The model under review builds one solid part; all positions refer to its coordinate system, in mm. A direction names the side the tool comes from. Coordinates: 2 decimals unless noted, no trailing zeros. Loops run counter-clockwise (first coordinate to the right, second up) from the corner with the lowest first, then second, coordinate; pieces in that order, holes last. Notation, with made-up numbers: M -9,12 L 42,12 A15 ccw 42,32 Z; hole C -4.75,-14.5 d1. An arc over 180 degrees is marked long. Write item = value, one per line. Start each with the question number.
Q1. For faces 5 (the face through (6.847, -0.766, -6.591)), 6 (the face through (3, 0, 0)), 7 (the face through (-5, 0, 5)), 8 (the face through (40, -5, -2)), 9 (the face through (-5, 0, -5)), list the 3-axis set-ups (+Z, -Z, +X, -X, +Y, -Y) from which the entire face can be reached by the end or side of a thin tool; tool diameter is ignored.
Q2. Mouldability with a two-part tool opening along Y and no side actions: class faces 1 (the face through (39.01, -4.88, 1.08)), 2 (the face through (19.72, -2.87, -6.93)), 3 (the face through (0, 2, 2)), 4 (the face through (38, 4, 4)) as released by +Y, released by -Y, zero draft, split by the parting line, or undercut.
Q3. Clearance check with flat-ended pins moving along their axes: pin 1 Ø1 at (x, y) = (16, -1) entering from -Z; pin 2 Ø5.5 at (x, y) = (-5.5, -1) entering from +Z; pin 3 Ø4 at (x, y) = (-5.5, -1) entering from -Z. State where each tip first meets the part, or that it passes through.
Q4. We need section A-A on y = 1.25. Give the boundary of the cut face in (x, z), and give its area (3 significant figures).
Q5. We need section D-D on x = 14. Give the boundary of the cut face in (y, z), and give its area (3 significant figures).
Q6. Wall thickness on probe 1 along X at (y, z) = (5, 2.5); probe 2 along Y at (x, z) = (38.75, 0); probe 3 along X at (y, z) = (-3.25, 6.25): over which ranges is each line inside the solid? List them lowest first.
Q7. We need section B-B on x = 5. Give the boundary of the cut face in (y, z).
Q8. We need section C-C on z = 0. Give the boundary of the cut face in (x, y), and give its area (3 significant figures).
from build123d import *

# Parameters (mm, degrees)
SKETCH1_R                = 7.5
BOSS_EXTRUDE1_DEPTH      = 40
SKETCH2_R                = 5
CUT_EXTRUDE1_DEPTH       = 2
SKETCH3_R                = 6
CUT_EXTRUDE2_DEPTH       = 35
SKETCH4_R                = 2.5
BOSS_EXTRUDE4_DEPTH      = 5
BOSS_EXTRUDE5_DEPTH      = 5
BOSS_EXTRUDE5_DEPTH_BACK = 5
SKETCH6_R                = 2.5
CUT_EXTRUDE3_START       = -7.500000101
CUT_EXTRUDE3_OUTLINE_R   = 2
CUT_EXTRUDE3_DEPTH       = 15.000000201


# Read off the part's stored shape, not the designer's step: Cut-Extrude3
with BuildPart() as part:
    # Sketch1 → Boss-Extrude1 (new body)
    with BuildSketch(Plane(origin=(0, 0, 0), x_dir=(0, 0, -1), z_dir=(1, 0, 0))):
        Circle(SKETCH1_R)
    extrude(amount=BOSS_EXTRUDE1_DEPTH)

    # Sketch2 → Cut-Extrude1 (cut)
    with BuildSketch(Plane(origin=(40, 0, 0), x_dir=(0, 0, -1), z_dir=(1, 0, 0))):
        Circle(SKETCH2_R)
    extrude(amount=-CUT_EXTRUDE1_DEPTH, mode=Mode.SUBTRACT)

    # Sketch3 → Cut-Extrude2 (cut)
    with BuildSketch(Plane(origin=(38, 0, 0), x_dir=(0, 0, -1), z_dir=(1, 0, 0))):
        Circle(SKETCH3_R)
    extrude(amount=-CUT_EXTRUDE2_DEPTH, mode=Mode.SUBTRACT)

    # Sketch4 → Boss-Extrude4 (add)
    with BuildSketch(Plane.ZY):
        with Locations(Location((0, 0, 0), (0, 0, 180))):
            Circle(SKETCH4_R)
    extrude(amount=BOSS_EXTRUDE4_DEPTH)

    # Sketch6 → Boss-Extrude5 (add, two sides: drawn at the far end of the back side and taken through both)
    with BuildSketch(Plane.XY.offset(-BOSS_EXTRUDE5_DEPTH_BACK)):
        with Locations((-5, 0)):
            Circle(SKETCH6_R)
    extrude(amount=BOSS_EXTRUDE5_DEPTH + BOSS_EXTRUDE5_DEPTH_BACK)

    # Cut-Extrude3 outline → Cut-Extrude3 (cut)
    with BuildSketch(Plane.XY.offset(CUT_EXTRUDE3_START)):
        with Locations((5, 0)):
            Circle(CUT_EXTRUDE3_OUTLINE_R)
    extrude(amount=CUT_EXTRUDE3_DEPTH, mode=Mode.SUBTRACT)


solid = part.part
Returned:
q1.face_5 = +Z, -Z
q1.face_6 = none
q1.face_7 = +Z, -X, +Y, -Y
q1.face_8 = +Z, -Z, +X, +Y, -Y
q1.face_9 = -Z, -X, +Y, -Y
q2.face_1 = undercut
q2.face_2 = split by the parting line
q2.face_3 = zero draft
q2.face_4 = undercut
q3.pin_1 = -7.48
q3.pin_2 = 5
q3.pin_3 = -5
q4.outline = M -7.17,-5 L -2.83,-5 L -2.83,-2.17 L 0,-2.17 L 0,-7.4 L 3.44,-7.4 L 3.44,-5.87 L 3,-5.87 L 3,5.87 L 3.44,5.87 L 3.44,7.4 L 0,7.4 L 0,2.17 L -2.83,2.17 L -2.83,5 L -7.17,5 Z; M 6.56,-7.4 L 40,-7.4 L 40,-4.84 L 38,-4.84 L 38,-5.87 L 6.56,-5.87 Z; M 6.56,5.87 L 38,5.87 L 38,4.84 L 40,4.84 L 40,7.4 L 6.56,7.4 Z
q4.area = 208 mm^2
q5.outline = C 0,0 d15; hole C 0,0 d12
q5.area = 63.6 mm^2
q6.probe_1 = 0 to 3, 38 to 40
q6.probe_2 = -7.5 to -5, 5 to 7.5
q6.probe_3 = 0 to 40
q7.outline = M -2,-7.23 L -2,-5.66 A6 cw -2,5.66 L -2,7.23 A7.5 ccw Z; M 2,-7.23 A7.5 ccw 2,7.23 L 2,5.66 A6 cw 2,-5.66 Z
q8.outline = M -5,-2.5 L 0,-2.5 L 0,-7.5 L 40,-7.5 L 40,-5 L 38,-5 L 38,-6 L 3,-6 L 3,6 L 38,6 L 38,5 L 40,5 L 40,7.5 L 0,7.5 L 0,2.5 L -5,2.5 A2.5 ccw Z
q8.area = 195 mm^2
